Check sheet for the modelled part. Datum: model origin and axes. Units: mm. A direction names the side the tool comes from. Round coordinates to 2 decimals unless told otherwise and drop trailing zeros. Write each loop counter-clockwise with the first axis right and the second up, starting at its lowest first coordinate (ties: lowest second). Pieces come first, ordered by that corner, then holes. Notation, with made-up numbers: (18.25, -18.75) -> (29.25, -18.75) arc R19 ccw to (29.25, -10.75) -> close; hole circle Ø8 at (18, -17.5). An arc over 180 degrees is marked (long way). Answer as a JSON object with one key per item and string values. Group by question number.
```python
from build123d import *

# Parameters (mm, degrees)
SKETCH_R  = 5
PAD_DEPTH = 2


with BuildPart() as part:
    # Sketch → Pad (new body)
    with BuildSketch(Plane.XY):
        with BuildLine():
            Line((-22.506098, 36), (45.373485, 36))
            ThreePointArc((61.217774, 17.77323), (57.448838, 30.496944), (45.373485, 36))
            Line((61.217774, 17.77323), (52.902681, -41.391731))
            ThreePointArc((33.68459, -43.636364), (44.160093, -49.932481), (52.902681, -41.391731))
            ThreePointArc((33.68459, -43.636364), (29.275011, -38.091326), (22.506098, -36))
            Line((22.506098, -36), (-37, -36))
            ThreePointArc((-53, -20), (-48.313708, -31.313708), (-37, -36))
            Line((-53, -20), (-53, 40))
            ThreePointArc((-33.68459, 43.636364), (-44.850122, 49.827362), (-53, 40))
            ThreePointArc((-33.68459, 43.636364), (-29.275011, 38.091326), (-22.506098, 36))
        make_face()
        with Locations((-43, 40)):
            Circle(SKETCH_R, mode=Mode.SUBTRACT)
        with Locations((43, -40)):
            Circle(SKETCH_R, mode=Mode.SUBTRACT)
        with BuildLine():
            Line((-35, 30), (45.373485, 30))
            ThreePointArc((55.276165, 18.608269), (52.92058, 26.56059), (45.373485, 30))
            Line((55.276165, 18.608269), (51.348271, -9.340154))
            ThreePointArc((27.581837, -30), (43.327254, -24.11303), (51.348271, -9.340154))
            Line((27.581837, -30), (-37, -30))
            ThreePointArc((-47, -20), (-44.071068, -27.071068), (-37, -30))
            Line((-47, -20), (-47, 18))
            ThreePointArc((-35, 30), (-43.485281, 26.485281), (-47, 18))
        make_face(mode=Mode.SUBTRACT)
    extrude(amount=PAD_DEPTH)


solid = part.part
```
(1) Section check C-C on x = 7.5. Record the cut outline in (y, z).
(2) Scan lines: line 1 along Y through (x, z) = (43, 1.2); line 2 along Y through (x, z) = (1.5, 0.1); line 3 along Y through (x, z) = (-44, 1.95). Record each from-to range of solid material in increasing order.
(3) Section check D-D on x = 43. Record the cut outline in (y, z), then the cut area to 3 significant figures.
(4) Access from +Z, -Z, +X, -X, +Y, -Y to the whole of each face (thin tool, end or side, straight path). Record for faces 5 (the flat face through (53.34, 4.83, 0.99)), 6 (the flat face through (57.118, -11.395, 0.986)).
(5) Section check A-A on z = 1.05. Record the cut outline in (x, y).
(6) Release check for a two-part mould opening along X. For faces 1 (the cylindrical face through (-29.36, 38.15, 0.99)), 2 (the flat face through (9, 34, 2)), 3 (the cylindrical face through (43.98, -49.95, 0.99)), 4 (the cylindrical face through (-47, 43, 1)) record: pulls with the +X half, pulls with the -X half, needs draft (parallel to the pull), parting line crosses it, or undercut.
(7) Section check B-B on y = 20.5. Record the cut outline in (x, z).
(8) Go/stop test with flat-tipped pins: pin 1 Ø13 at (x, y) = (-43, 40) entering from +Z; pin 2 Ø0.6 at (x, z) = (-6, 0.5) entering from -Y; pin 3 Ø1 at (x, z) = (25, 1) entering from -Y. Record where each tip stops, or that it passes through.
Data:
{
 "1": {"outline": "(-36, 0) -> (-30, 0) -> (-30, 2) -> (-36, 2) -> close; (30, 0) -> (36, 0) -> (36, 2) -> (30, 2) -> close"},
 "2": {"line 1": "y = -50 to -45, -35 to -24.39, 30 to 36", "line 2": "y = -36 to -30, 30 to 36", "line 3": "y = -34.39 to -27.14, 25.94 to 35.1, 44.9 to 49.95"},
 "3": {"outline": "(-50, 0) -> (-45, 0) -> (-45, 2) -> (-50, 2) -> close; (-35, 0) -> (-24.39, 0) -> (-24.39, 2) -> (-35, 2) -> close; (30, 0) -> (36, 0) -> (36, 2) -> (30, 2) -> close", "area": "43.2 mm²"},
 "4": {"face 5": "+Z, -Z", "face 6": "+Z, -Z, +X, -Y"},
 "5": {"outline": "(-53, -20) arc R16 ccw to (-37, -36) -> (22.51, -36) arc R12 cw to (33.68, -43.64) arc R10 ccw to (52.9, -41.39) -> (61.22, 17.77) arc R16 ccw to (45.37, 36) -> (-22.51, 36) arc R12 cw to (-33.68, 43.64) arc R10 ccw to (-53, 40) -> close; hole circle Ø10 at (-43, 40); hole (-47, -20) arc R10 ccw to (-37, -30) -> (27.58, -30) arc R24 ccw to (51.35, -9.34) -> (55.28, 18.61) arc R10 ccw to (45.37, 30) -> (-35, 30) arc R12 ccw to (-47, 18) -> close; hole circle Ø10 at (43, -40)"},
 "6": {"face 1": "pulls with the +X half", "face 2": "needs draft", "face 3": "parting line crosses it", "face 4": "undercut"},
 "7": {"outline": "(-53, 0) -> (-46.74, 0) -> (-46.74, 2) -> (-53, 2) -> close; (55.36, 0) -> (61.37, 0) -> (61.37, 2) -> (55.36, 2) -> close"},
 "8": {"pin 1": "stops at z = 2", "pin 2": "stops at y = -36", "pin 3": "stops at y = -36.38"}
}
